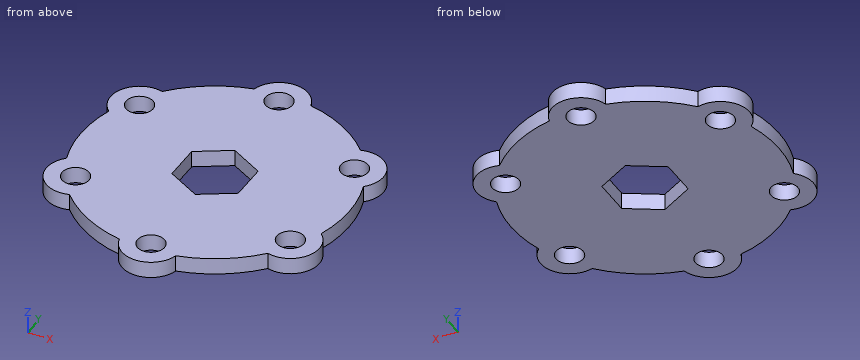
Autodesk Inventor part; units mm, degrees
ref_plane "YZ Plane" through (0, 0, 0) normal (1, 0, 0) x (0, 1, 0)
ref_plane "XZ Plane" through (0, 0, 0) normal (0, 1, 0) x (-1, 0, 0)
ref_plane "XY Plane" through (0, 0, 0) normal (0, 0, 1) x (1, 0, 0)
sketch "Sketch1" plane through (0, 0, 0) normal (0, 0, 1) x (1, 0, 0)
  circle A0 centre (0, 0) radius 28.575
  line L0 (0, -7.3617) -> (6.3754, -3.6809)
  line L1 (-6.3754, -3.6809) -> (0, -7.3617)
  line L2 (-6.3754, 3.6808) -> (-6.3754, -3.6809)
  line L3 (0, 7.3617) -> (-6.3754, 3.6808)
  line L4 (6.3754, 3.6808) -> (0, 7.3617)
  line L5 (6.3754, -3.6809) -> (6.3754, 3.6808)
  circle A1 centre (0, 23.8125) radius 2.5908
  circle A2 centre (-20.6222, 11.9062) radius 2.5908
  circle A3 centre (-20.6222, -11.9062) radius 2.5908
  circle A4 centre (0, -23.8125) radius 2.5908
  circle A5 centre (20.6222, -11.9063) radius 2.5908
  circle A6 centre (20.6222, 11.9062) radius 2.5908
  arc A7 (-2.587, 23.6716) -> (-19.2067, 14.0762) centre (0, 0) ccw
  arc A8 (-21.7937, 9.5954) -> (-21.7937, -9.5954) centre (0, 0) ccw
  arc A9 (-19.2067, -14.0762) -> (-2.587, -23.6716) centre (0, 0) ccw
  arc A10 (2.587, -23.6716) -> (19.2067, -14.0762) centre (0, 0) ccw
  arc A11 (21.7937, -9.5954) -> (21.7937, 9.5954) centre (0, 0) ccw
  arc A12 (19.2067, 14.0762) -> (2.587, 23.6716) centre (0, 0) ccw
  dimension "d7" = 5.1816
  dimension "d12" = 360
extrude "Extrusion1" add sketch "Sketch1" along normal blind 3.175 contours A0 | A1 A12 A6 A11 A5 A10 A4 A9 A3 A8 A2 A7
sketch "Sketch3" plane through (0, 0, 3.175) normal (0, 0, 1) x (1, 0, 0)
  circle A0 centre (20.6222, 11.9062) radius 2.5908
  circle A1 centre (20.6222, -11.9063) radius 2.5908
  circle A2 centre (0, -23.8125) radius 2.5908
  circle A3 centre (-20.6222, -11.9062) radius 2.5908
  circle A4 centre (-20.6222, 11.9062) radius 2.5908
  circle A5 centre (0, 23.8125) radius 2.5908
  circle A6 centre (0, 0) radius 28.575
  circle A7 centre (0, 23.8125) radius 5.5626
  circle A8 centre (0, 0) radius 25.6794
  circle A9 centre (-20.6222, 11.9062) radius 5.5626
  circle A10 centre (-20.6222, -11.9062) radius 5.5626
  circle A11 centre (0, -23.8125) radius 5.5626
  circle A12 centre (20.6222, -11.9063) radius 5.5626
  circle A13 centre (20.6222, 11.9062) radius 5.5626
  dimension "d14" = 11.1252
  dimension "d15" = 51.3588
  dimension "d18" = 360
extrude "Extrusion3" cut sketch "Sketch3" against normal blind 3.175 contours A0 A8 A13 A6 | A8 A7 A6 A13 | A13 A6 A12 A8 | A8 A5 A7 A6 | A12 A6 A8 A1 | A8 A9 A6 A7 | A12 A6 A11 A8 | A8 A4 A9 A6 | A11 A6 A8 A2 | A9 A8 A10 A6 | A10 A8 A3 A6 | A6 A10 A8 A11
extrude "Extrusion2" add sketch "Sketch3" against normal blind 3.175 contours A0 A8 A13 A6 | A0 A8 A13 | A8 A5 A7 A6 | A7 A8 A5 | A13 A6 | A6 A7 | A12 A6 A8 A1 | A8 A1 A12 | A12 A6 | A9 A8 A4 | A8 A4 A9 A6 | A6 A9 | A11 A6 A8 A2 | A8 A2 A11 | A11 A6 | A10 A8 A3 A6 | A6 A10 | A10 A8 A3
properties part number "chassis hex hub clone" material "Aluminum 6061"
Input: part model. Units: mm. Frame: model coordinates. Round coordinates to 2 decimals unless told otherwise and drop trailing zeros. Write each loop counter-clockwise with the first axis right and the second up, starting at its lowest first coordinate (ties: lowest second). Pieces come first, ordered by that corner, then holes. Notation, with made-up numbers: (52, 60) - (56, 60) arc R18 cw to (56, 87) - close; hole circle Ø1 at (75.25, 40.25). An arc over 180 degrees is marked (long way). Write item = value, one per line.
(1) Section query D-D on x = -16. Output: boundary loops of the cut face in (y, z) (3 decimals), then the cut area to 3 significant figures.
Geometry check:
outline = (-20.086, 0) - (20.086, 0) - (20.086, 3.175) - (-20.086, 3.175) - close
area = 128 mm^2
(2) Section query A-A on x = 4. Output: boundary loops of the cut face in (y, z) (3 decimals), then the cut area to 3 significant figures.
Geometry check:
outline = (-27.678, 0) - (-5.052, 0) - (-5.052, 3.175) - (-27.678, 3.175) - close; (5.052, 0) - (27.678, 0) - (27.678, 3.175) - (5.052, 3.175) - close
area = 144 mm^2
(3) Material intervals for probe 1 along Y at (x, z) = (0, 0.9); probe 2 along X at (y, z) = (12, 1.3); probe 3 along X at (y, z) = (10, 0.65), sorted ascending.
Geometry check:
probe_1 = -29.38 to -26.4, -21.22 to -7.36, 7.36 to 21.22, 26.4 to 29.38
probe_2 = -26.18 to -23.21, -18.03 to 18.03, 23.21 to 26.18
probe_3 = -25.85 to -22.38, -18.87 to 18.87, 22.38 to 25.85
(4) Contact query for flat-ended pins moving along their axis: pin 1 Ø3 at (x, y) = (0, 23.81) entering from -Z; pin 2 Ø1.6 at (y, z) = (-1.5, 2) entering from +X; pin 3 Ø1 at (x, z) = (13.5, 1) entering from -Y; pin 4 Ø1.6 at (y, z) = (2, 1.5) entering from -X. Output: stop coordinate, or through.
Geometry check:
pin_1 = through
pin_2 = 25.67
pin_3 = -22.15
pin_4 = -25.65
(5) Section query C-C on z = 0.75. Output: boundary loops of the cut face in (x, y), then the cut area to 3 significant figures.
Geometry check:
outline = (-24.45, -7.87) arc R5.56 ccw to (-19.03, -17.24) arc R25.68 ccw to (-5.41, -25.1) arc R5.56 ccw to (5.41, -25.1) arc R25.68 ccw to (19.03, -17.24) arc R5.56 ccw to (24.45, -7.87) arc R25.68 ccw to (24.45, 7.87) arc R5.56 ccw to (19.03, 17.24) arc R25.68 ccw to (5.41, 25.1) arc R5.56 ccw to (-5.41, 25.1) arc R25.68 ccw to (-19.03, 17.24) arc R5.56 ccw to (-24.45, 7.87) arc R25.68 ccw to start; hole circle Ø5.18 at (-20.62, -11.91); hole circle Ø5.18 at (-20.62, 11.91); hole (-6.38, -3.68) - (0, -7.36) - (6.38, -3.68) - (6.38, 3.68) - (0, 7.36) - (-6.38, 3.68) - close; hole circle Ø5.18 at (0, -23.81); hole circle Ø5.18 at (0, 23.81); hole circle Ø5.18 at (20.62, -11.91); hole circle Ø5.18 at (20.62, 11.91)
area = 1,990 mm^2
(6) Section query B-B on y = -4.5. Output: boundary loops of the cut face in (x, z) (3 decimals), then the cut area to 3 significant figures.
Geometry check:
outline = (-25.282, 0) - (-4.957, 0) - (-4.957, 3.175) - (-25.282, 3.175) - close; (4.957, 0) - (25.282, 0) - (25.282, 3.175) - (4.957, 3.175) - close
area = 129 mm^2
